Source: CAD feature listing. Evaluate the final solid. Frame: model axes, mm. A direction names the side the tool comes from. Give positions to 0.01 mm unless a question says otherwise; leave off trailing zeros. Loops run counter-clockwise (first coordinate to the right, second up) from the corner with the lowest first, then second, coordinate; pieces in that order, holes last. Notation, with made-up numbers: (65, 7) - (122, 7) arc R8 cw to (122, 16) - close; hole circle Ø4 at (36.25, 20). An arc over 180 degrees is marked (long way). Write each question's results on one line, items separated by ' | '. Start each with the question number.
(1) Contact query for flat-ended pins moving along their axis: pin 1 (3.5 mm diameter, centred on x = 2, y = 66.5, fed in from +Z); pin 2 (22.5 mm diameter, centred on y = 32, z = 27.5, fed in from +X); pin 3 (8.5 mm diameter, centred on x = 42, y = 18, fed in from +Z); pin 4 (5.5 mm diameter, centred on x = 18, y = 42, fed in from +Z). Output: stop coordinate, or through.
(2) Cut plane D-D on y = 50. Return the cut outline in (x, z).
(3) Cut plane A-A on x = 69. Return the cut outline in (y, z), then the cut area to 3 significant figures.
(4) Reachability of faces 1 (the cylindrical face through (18.43, 65.73, 1.52)), 2 (the flat face through (33, 67, 1)), 3 (the flat face through (33, 3, 34)), 4 (the flat face through (1, 33, 67)), 5 (the cylindrical face through (33.444, 1.521, 58.22)) from +Z, -Z, +X, -X, +Y, -Y: full face, straight path, thin tool, end or side. Return the list, or none.
(5) Cut plane C-C on x = 47.5. Return the cut outline in (y, z).
(6) Material intervals for line 1 along Y through (x, z) = (18, 1.6); line 2 along Y through (x, z) = (18, 1.1); line 3 along X through (y, z) = (11.5, 52.5), sorted ascending. Write a range as [from, to].
(7) Pull-direction query (Y, two-part tool) for faces 6 (the cylindrical face through (58.22, 33.444, 1.521)), 7 (the cylindrical face through (78.289, 1.521, 31.196)), 8 (the cylindrical face through (1.479, 44.619, 15.992)); classes: pulls with the +Y half, pulls with the -Y half, needs draft (parallel to the pull), parting line crosses it, or undercut.
from build123d import *

# Parameters (mm, degrees)
F1_DEPTH = 3
F3_DEPTH = 3
F5_DEPTH = 3
F7_D     = 6.6
F9_D     = 6.6
F11_D    = 6.6
F12_R    = 6
F13_R    = 1.5


with BuildPart() as f1:
    # F0 (on Front) → F1 (new body)
    with BuildSketch(Plane.XZ):
        Polygon((33, 80), (0, 80), (0, 0), (80, 0), (80, 33), (58, 33), (33, 58), align=None)
    extrude(amount=-F1_DEPTH)

    # F2 (on Right) → F3 (join)
    with BuildSketch(Plane.YZ):
        Polygon((0, 80), (0, 0), (80, 0), (80, 33), (58, 33), (33, 58), (33, 80), align=None)
    extrude(amount=F3_DEPTH)

    # F4 (on face) → F5 (join)
    with BuildSketch(Plane(origin=(0, 0, 0), x_dir=(1, 0, 0), z_dir=(0, 0, -1))):
        Polygon((80, 0), (0, 0), (0, -80), (33, -80), (33, -58), (58, -33), (80, -33), align=None)
    extrude(amount=-F5_DEPTH)

    # F7 (through all)
    with Locations(Plane.XZ):
        with Locations((42, 18), (69, 18), (18, 69), (18, 42)):
            Hole(F7_D / 2)

    # F9 (through all)
    with Locations(Plane.YZ.offset(3)):
        with Locations((42, 18), (69, 18), (18, 69), (18, 42)):
            Hole(F9_D / 2)

    # F11 (through all)
    with Locations(Plane(origin=(0, 0, 0), x_dir=(1, 0, 0), z_dir=(0, 0, -1))):
        with Locations((42, -18), (69, -18), (18, -42), (18, -69)):
            Hole(F11_D / 2)

    # F12
    f12_edges = [f1.edges().sort_by_distance(p)[0] for p in [
        (33, 1.5, 80),
        (1.5, 80, 33),
        (80, 1.5, 33),
        (33, 1.5, 58),
        (58, 1.5, 33),
        (58, 33, 1.5),
        (33, 58, 1.5),
        (1.5, 58, 33),
        (1.5, 33, 58),
        (1.5, 33, 80),
        (33, 80, 1.5),
        (80, 33, 1.5),
    ]]
    fillet(f12_edges, radius=F12_R)

    # F13
    f13_edges = [f1.edges().sort_by_distance(p)[0] for p in [
        (41.5, 3, 3),
        (3, 41.5, 3),
        (3, 3, 41.5),
        (40, 0, 0),
        (0, 0, 40),
        (0, 40, 0),
    ]]
    fillet(f13_edges, radius=F13_R)


solid = f1.part
Ans:
1) pin 1: z = 33 | pin 2: x = 3 | pin 3: z = 3 | pin 4: through
2) outline: (0, 1.5) arc R1.5 ccw to (1.5, 0) - (41, 0) - (41, 3) - (4.5, 3) arc R1.5 cw to (3, 4.5) - (3, 41) - (0, 41) - close
3) outline: (0, 1.5) arc R1.5 ccw to (1.5, 0) - (14.7, 0) - (14.7, 3) - (4.5, 3) arc R1.5 cw to (3, 4.5) - (3, 14.7) - (0, 14.7) - close; (0, 21.3) - (3, 21.3) - (3, 33) - (0, 33) - close; (21.3, 0) - (33, 0) - (33, 3) - (21.3, 3) - close | area: 149 mm^2
4) face 1: +Z, -Z | face 2: +Z, -Z, +X, +Y | face 3: +Z, +X, +Y | face 4: +Z, +X, -X, +Y | face 5: +Z, +X, +Y, -Y
5) outline: (0, 1.5) arc R1.5 ccw to (1.5, 0) - (43.5, 0) - (43.5, 3) - (4.5, 3) arc R1.5 cw to (3, 4.5) - (3, 43.5) - (0, 43.5) - close
6) line 1: [0, 38.7], [45.3, 65.7], [72.3, 80] | line 2: [0.05, 38.7], [45.3, 65.7], [72.3, 80] | line 3: [0, 3]
7) face 6: pulls with the +Y half | face 7: needs draft | face 8: undercut
